The listing builds one solid part. Answer for the finished solid, in the listing's coordinates (mm). Face numbers are marked on the shaded views. A direction names the side the tool comes from. Give positions to 0.01 mm unless a question says otherwise; leave off trailing zeros. Write each loop counter-clockwise with the first axis right and the second up, starting at its lowest first coordinate (ties: lowest second). Pieces come first, ordered by that corner, then holes. Notation, with made-up numbers: (26.5, 31) - (49.5, 31) arc R20 cw to (49.5, 67) - close; hole circle Ø1 at (61, -3.75). An arc over 180 degrees is marked (long way). One line per question, with ' | ' between items. Start each with the question number.
1. Given P1, Ø1.3, axis at y = -1.5, z = 2.5, coming from the +X side; P2, Ø0.9, axis at x = 3, z = 3, coming from the -Y side; P3, Ø0.8, axis at y = -1.5, z = 2.5, coming from the -X side, each flat-ended and moving along its own axis, determine where each tip first touches the part or whether it passes through.
2. A cutting plane is placed at D-D (x = 14.25). Determine the outline of the cut face in (y, z).
3. For the marked faces 1, 2, 3 and 4, determine the directions among +Z, -Z, +X, -X, +Y, -Y from which every point of the face is accessible in a straight line to the end or side of a thin tool.
4. A cutting plane is placed at A-A (z = 3.25). Determine the outline of the cut face in (x, y), then the cut area to 3 significant figures.
5. Find the intervals of material crossed by L1, parallel to X at y = -0.7, z = 1.6; L2, parallel to Z at x = 17.75, y = -3.3; L3, parallel to Y at x = 2.5, z = 2.3, in increasing order. Write a range as from..to.
6. A cutting plane is placed at C-C (x = 3). Determine the outline of the cut face in (y, z).
7. A cutting plane is placed at B-B (y = -1.9). Determine the outline of the cut face in (x, z), then the cut area to 3 significant figures.
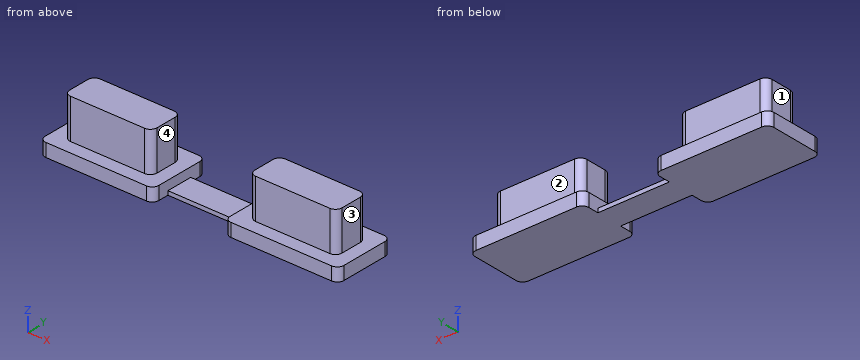
Autodesk Fusion 360 part; units mm, degrees
sketch "草图1" plane through (0, 0, 0) normal (0, 0, 1) x (1, 0, 0)
  line L0 (20.6, 0) -> (20.6, -2.6)
  line L1 (0, -2.6) -> (0, 0)
  line L2 (6.6, 0) -> (6.6, -2.6)
  line L3 (14, 0) -> (14, -2.6)
  line L4 (0, 0) -> (6.6, 0)
  line L5 (14, 0) -> (20.6, 0)
  line L6 (20.6, -2.6) -> (14, -2.6)
  line L7 (6.6, -2.6) -> (0, -2.6)
  line L8 (7.6, -3.6) -> (-1, -3.6)
  line L9 (-1, -3.6) -> (-1, 1)
  line L10 (-1, 1) -> (7.6, 1)
  line L11 (7.6, 1) -> (7.6, -3.6)
  line L12 (21.6, -3.6) -> (13, -3.6)
  line L13 (13, 1) -> (13, -3.6)
  line L14 (13, 1) -> (21.6, 1)
  line L15 (21.6, 1) -> (21.6, -3.6)
  line L16 (7.6, -0.3) -> (13, -0.3)
  line L17 (7.6, -2.3) -> (13, -2.3)
  dimension "d2" = 2.6
  dimension "d3" = 6.6
  dimension "d4" = 6.6
  dimension "d7" = -1
  dimension "d8" = -1
  dimension "d9" = 2
  dimension "d10" = 0.3
  dimension "d19" = 5.4
extrude "拉伸1" add sketch "草图1" along normal blind 1 contours L0 L3 L5 L6 | L1 L2 L4 L7 | L8 L9 L10 L11 | L12 L13 L14 L15 makes body 1 at (1.8667, -0.5333, 0) makes body 2 at (15.8667, -0.5333, 0)
extrude "拉伸2" add sketch "草图1" along normal blind 0.3 contours L11 L13 L16 L17 bodies 1 2
extrude "拉伸3" add sketch "草图1" along normal blind 4 contours L0 L3 L5 L6 | L1 L2 L4 L7 bodies 1
fillet "圆角1" radius 0.5 16 edges at (6.6, -2.6, 2.5) (6.6, 0, 2.5) (0, 0, 2.5) (0, -2.6, 2.5) (-1, -3.6, 0.5) (-1, 1, 0.5) (7.6, 1, 0.5) (7.6, -3.6, 0.5) (14, -2.6, 2.5) (13, -3.6, 0.5) (13, 1, 0.5) (21.6, -3.6, 0.5) (21.6, 1, 0.5) (20.6, 0, 2.5) (20.6, -2.6, 2.5) (14, 0, 2.5) on bodies 1
Determined:
1) P1: x = 20.6 | P2: y = -2.6 | P3: x = 0
2) outline: (-3.6, 0) - (1, 0) - (1, 1) - (-0.07, 1) - (-0.07, 4) - (-2.53, 4) - (-2.53, 1) - (-3.6, 1) - close
3) face 1: +Z, -X, +Y, -Y | face 2: +Z, +X, -X, +Y | face 3: +Z, +X, +Y, -Y | face 4: +Z, +Y, -Y
4) outline: (0, -2.1) arc R0.5 ccw to (0.5, -2.6) - (6.1, -2.6) arc R0.5 ccw to (6.6, -2.1) - (6.6, -0.5) arc R0.5 ccw to (6.1, 0) - (0.5, 0) arc R0.5 ccw to (0, -0.5) - close; (14, -2.1) arc R0.5 ccw to (14.5, -2.6) - (20.1, -2.6) arc R0.5 ccw to (20.6, -2.1) - (20.6, -0.5) arc R0.5 ccw to (20.1, 0) - (14.5, 0) arc R0.5 ccw to (14, -0.5) - close | area: 33.9 mm2
5) L1: 0..6.6, 14..20.6 | L2: 0..1 | L3: -2.6..0
6) outline: (-3.6, 0) - (1, 0) - (1, 1) - (0, 1) - (0, 4) - (-2.6, 4) - (-2.6, 1) - (-3.6, 1) - close
7) outline: (-1, 0) - (21.6, 0) - (21.6, 1) - (20.6, 1) - (20.6, 4) - (14, 4) - (14, 1) - (13, 1) - (13, 0.3) - (7.6, 0.3) - (7.6, 1) - (6.6, 1) - (6.6, 4) - (0, 4) - (0, 1) - (-1, 1) - close | area: 58.4 mm2
